Part model, mm, in its own coordinate system. A direction names the side the tool comes from. Round coordinates to 2 decimals unless told otherwise and drop trailing zeros. Order: outer loops, then holes, each group sorted by start corner. A loop starts at its lowest first (then second) coordinate and runs counter-clockwise, first axis right, second up. Notation, with made-up numbers: (33.5, 41) - (56.5, 41) arc R23 cw to (56.5, 59) - close; hole circle Ø3 at (65, -22.75). An arc over 180 degrees is marked (long way). Answer as a JSON object with one key per item and string values.
```python
from build123d import *

# Parameters (mm, degrees)
F0_R      = 16.6957172427
F1_DEPTH  = 62.738
F2_W      = 33.8111482561
F2_H      = 95.895409584
F3_DEPTH  = 62.738
F4_R      = 13.2741365626
F5_DEPTH  = 55.372
F6_W      = 12.5334430486
F6_H      = 82.7790144831
F7_DEPTH  = 55.372
F8_R      = 15.0046147667
F9_DEPTH  = 49.022
F10_W     = 14.5737715065
F10_H     = 64.1245916486
F11_DEPTH = 49.022
F13_DEPTH = 4.826
F14_W     = 4.4474024326
F14_H     = 8.5983164608
F15_DEPTH = 76.962
F16_W     = 50.9968847036
F16_H     = 3.2614283264
F17_DEPTH = 72.644
F18_W     = 10.0807789713
F18_H     = 3.5579204559
F19_DEPTH = 72.136
F20_W     = 55.1477968693
F20_H     = 17.4931138754
F21_DEPTH = 53.848


with BuildPart() as f1:
    # F0 (on Top) → F1 (new body)
    with BuildSketch(Plane.XY):
        with Locations((9.0357372537, 35.1227857172)):
            Circle(F0_R)
    extrude(amount=F1_DEPTH)

    # F2 (on Top) → F3 (join)
    with BuildSketch(Plane.XY):
        with Locations((9.035738185, -16.0311460495)):
            Rectangle(F2_W, F2_H)
    extrude(amount=F3_DEPTH)

    # F4 (on Top) → F5 (join)
    with BuildSketch(Plane.XY):
        with Locations((-7.5783608481, 18.2375591248)):
            Circle(F4_R)
    extrude(amount=F5_DEPTH)

    # F6 (on Top) → F7 (join)
    with BuildSketch(Plane.XY):
        with Locations((-14.1365574673, -22.2775219008)):
            Rectangle(F6_W, F6_H)
    extrude(amount=F7_DEPTH)

    # F8 (on Top) → F9 (join)
    with BuildSketch(Plane.XY):
        with Locations((-20.2778875828, 3.7891804241)):
            Circle(F8_R)
    extrude(amount=F9_DEPTH)

    # F10 (on Top) → F11 (join)
    with BuildSketch(Plane.XY):
        with Locations((-27.8562474996, -32.0622958243)):
            Rectangle(F10_W, F10_H)
    extrude(amount=F11_DEPTH)

    # F12 (on Front) → F13 (join)
    with BuildSketch(Plane.XZ):
        with BuildLine():
            add(Edge.make_bspline(
                [(9.3272132799, 78.8237527013), (7.9182853633, 76.8284104093), (5.182542099, 72.9540147279), (6.7369025998, 66.8272809439), (2.8994250841, 61.239011136), (16.8173248262, 61.1527732675), (12.9666307345, 74.2246924308), (23.7803791476, 73.080684286), (18.3812111376, 62.4937182841), (23.573835168, 62.2986103244), (25.9413123131, 62.2096545994)],
                knots=[0, 0, 0, 0, 0.128166769, 0.248863956, 0.3478557526, 0.4875439615, 0.6364878053, 0.7485115106, 0.8853386559, 1, 1, 1, 1], degree=3))
            Line((25.9413123131, 62.2096545994), (25.9413123131, 78.8237527013))
            Line((25.9413123131, 78.8237527013), (9.3272132799, 78.8237527013))
        make_face()
    extrude(amount=F13_DEPTH)

    # F14 (on Top) → F15 (join)
    with BuildSketch(Plane.XY):
        with Locations((-28.3151315525, -60.6435146183)):
            Rectangle(F14_W, F14_H)
    extrude(amount=F15_DEPTH)

    # F16 (on Top) → F17 (join)
    with BuildSketch(Plane.XY):
        with Locations((-0.2964939922, -61.8294868618)):
            Rectangle(F16_W, F16_H)
    extrude(amount=F17_DEPTH)

    # F18 (on Top) → F19 (join)
    with BuildSketch(Plane.XY):
        with Locations((-35.5792222545, -62.2742250562)):
            Rectangle(F18_W, F18_H)
    extrude(amount=F19_DEPTH)

    # F20 (on Top) → F21 (join)
    with BuildSketch(Plane.XY):
        with Locations((-38.8406515121, -72.5032538176)):
            Rectangle(F20_W, F20_H)
    extrude(amount=F21_DEPTH)


solid = f1.part
```
Item 1: Cut at A-A (z = 57.5). Write the cut outline in (x, y), plus the area to 3 significant figures.
Taken from the geometry:
{"outline": "(-40.62, -64.05) - (-30.54, -64.05) - (-30.54, -64.94) - (-26.09, -64.94) - (-26.09, -56.34) - (-30.54, -56.34) - (-30.54, -60.5) - (-40.62, -60.5) - close; (-25.79, -63.46) - (-7.87, -63.46) - (-7.87, -63.98) - (25.94, -63.98) - (25.94, 31.92) - (25.42, 31.92) arc R16.7 ccw (long way) to (-7.35, 31.92) - (-7.87, 31.92) - (-7.87, -60.2) - (-25.79, -60.2) - close", "area": "3,920 mm2"}
Item 2: Drop flat-ended pins along their axis: P1, Ø8, axis at y = -27.5, z = 34.5, coming from the -X side; P2, Ø2, axis at x = 5.5, z = 69.5, coming from the +Y side; P3, Ø1.5, axis at x = -27, z = 18.5, coming from the +Y side. Give the stop position or say it passes through.
Taken from the geometry:
{"P1": "x = -35.14", "P2": "y = 0", "P3": "y = 17.55"}
Item 3: Cut at D-D (y = -7.5). Write the cut outline in (x, z), plus the area to 3 significant figures.
Taken from the geometry:
{"outline": "(-35.14, 0) - (25.94, 0) - (25.94, 62.74) - (-7.87, 62.74) - (-7.87, 55.37) - (-20.4, 55.37) - (-20.4, 49.02) - (-35.14, 49.02) - close", "area": "3,540 mm2"}
Item 4: Tool access for faces 4 (the flat face through (15, 0, 73)), 5 (the flat face through (-54, -63.757, 27)), 6 (the flat face through (25.941, -15, 30)), 7 (the flat face through (-26.091, -61, 63)), 8 (the flat face through (-36, -62, 72.136)): list every direction of +Z, -Z, +X, -X, +Y, -Y with a clear straight run to the whole face (end or side of a thin tool).
Taken from the geometry:
{"face 4": "+Z, +X, -X, +Y", "face 5": "+Z, -Z, -X, +Y", "face 6": "+Z, -Z, +X, +Y, -Y", "face 7": "+Z, +Y", "face 8": "+Z, -X, +Y, -Y"}
Item 5: Cut at B-B (y = -45). Write the cut outline in (x, z).
Taken from the geometry:
{"outline": "(-35.14, 0) - (-20.57, 0) - (-20.57, 49.02) - (-35.14, 49.02) - close; (-20.4, 0) - (25.94, 0) - (25.94, 62.74) - (-7.87, 62.74) - (-7.87, 55.37) - (-20.4, 55.37) - close"}
Item 6: Two-plate mould, pull along Y, no slides. Class faces 1 (the flat face through (-6, -60.199, 66)), 2 (the flat face through (-66.415, -73, 27)), 3 (the flat face through (-36, -64.053, 63)): pulls with the +Y half, pulls with the -Y half, needs draft (parallel to the pull), parting line crosses it, or undercut.
Taken from the geometry:
{"face 1": "undercut", "face 2": "needs draft", "face 3": "pulls with the -Y half"}
Item 7: Probe L1, parallel to X at y = -32, z = 40.5; L2, parallel to X at y = -9, z = 60; L3, parallel to Z at x = -32, y = -37. List the from-to ranges inside material, lowest first. Write a range as from..to.
Taken from the geometry:
{"L1": "-35.14..-20.57, -20.4..25.94", "L2": "-7.87..25.94", "L3": "0..49.02"}
Item 8: Cut at C-C (z = 12). Write the cut outline in (x, y), plus the area to 3 significant figures.
Taken from the geometry:
{"outline": "(-66.41, -81.25) - (-11.27, -81.25) - (-11.27, -63.76) - (-20.57, -63.76) - (-20.57, -63.46) - (-20.4, -63.46) - (-20.4, -63.67) - (-7.87, -63.67) - (-7.87, -63.98) - (25.94, -63.98) - (25.94, 31.92) - (25.42, 31.92) arc R16.7 ccw (long way) to (-7.35, 31.92) - (-7.87, 31.92) - (-7.87, 31.51) arc R13.27 ccw to (-20.84, 18.78) arc R15 ccw to (-34.8, 0) - (-35.14, 0) - (-35.14, -60.5) - (-40.62, -60.5) - (-40.62, -63.76) - (-66.41, -63.76) - close; hole (-20.57, -60.2) - (-20.4, -60.2) - (-20.4, -11.21) arc R15 cw to (-20.57, -11.21) - close", "area": "7,090 mm2"}
